Could you check a few things on this model? Use its own coordinates, in mm. Face numbers are marked on the shaded views. A direction names the side the tool comes from. Round coordinates to 2 decimals unless told otherwise and drop trailing zeros. Loops run counter-clockwise (first coordinate to the right, second up) from the corner with the lowest first, then second, coordinate; pieces in that order, holes last. Notation, with made-up numbers: (29, 39.25) -> (85, 39.25) arc R6 ccw to (85, 44.25) -> close; hole circle Ø2 at (55.25, 60.25). An arc over 180 degrees is marked (long way). One line per item, written item: value.
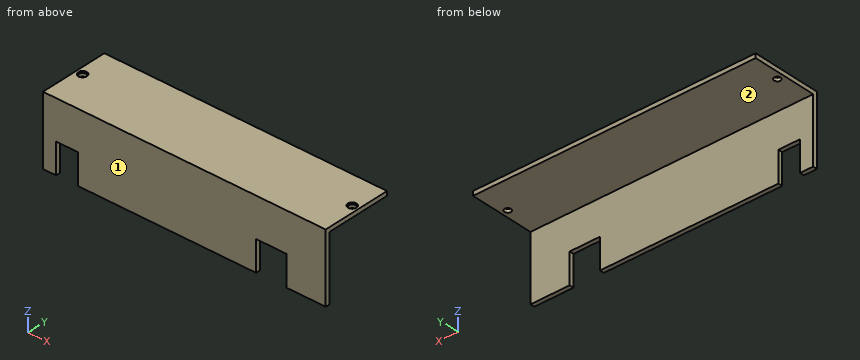
```python
from build123d import *

# Parameters (mm, degrees)
SKETCH021_W         = 130
SKETCH021_H         = 32
PAD009_DEPTH        = 2
HOLE005_D           = 3
HOLE005_DEPTH       = 25
HOLE005_CBORE_D     = 4
HOLE005_CBORE_DEPTH = 0.5
SKETCH023_W         = 130
SKETCH023_H         = 2
PAD010_DEPTH        = 30
SKETCH024_W         = 10
SKETCH024_H         = 15
SKETCH024_W_2       = 14
POCKET004_DEPTH     = 5


with BuildPart() as part:
    # Sketch021 → Pad009 (new body)
    with BuildSketch(Plane.XY.offset(31)):
        with Locations((65, -146.25)):
            Rectangle(SKETCH021_W, SKETCH021_H)
    extrude(amount=PAD009_DEPTH)

    # Hole005
    with Locations(Plane.XY.offset(33)):
        with Locations((3, -145), (127, -145)):
            CounterBoreHole(HOLE005_D / 2, HOLE005_CBORE_D / 2, HOLE005_CBORE_DEPTH, depth=HOLE005_DEPTH)

    # Sketch023 (on Face4 of Hole005) → Pad010 (join)
    with BuildSketch(Plane(origin=(0, 0, 31), x_dir=(1, 0, 0), z_dir=(0, 0, -1))):
        with Locations((65, 161.25)):
            Rectangle(SKETCH023_W, SKETCH023_H)
    extrude(amount=PAD010_DEPTH)

    # Sketch024 (on Face14 of Pad010) → Pocket004 (cut)
    with BuildSketch(Plane.XZ.offset(162.25)):
        with Locations((11, 7.5)):
            Rectangle(SKETCH024_W, SKETCH024_H)
        with Locations((105, 7.5)):
            Rectangle(SKETCH024_W_2, SKETCH024_H)
    extrude(amount=-POCKET004_DEPTH, mode=Mode.SUBTRACT)


solid = part.part
```
(1) On a 3-axis mill with a long thin cutter (end or side, diameter ignored), from which of +Z, -Z, +X, -X, +Y, -Y can I reach the whole of each face in a straight line? I mean the marked faces 1 and 2. Say none if no direction works.
Results below:
face 1: +Z, -Z, +X, -X, -Y
face 2: -Z, +X, -X, +Y
(2) Imagine slicing it at B-B on x = 127. Write out the boundary of the cut face in (y, z).
Results below:
outline: (-162.25, 1) -> (-160.25, 1) -> (-160.25, 31) -> (-146.5, 31) -> (-146.5, 32.5) -> (-147, 32.5) -> (-147, 33) -> (-162.25, 33) -> close; (-143.5, 31) -> (-130.25, 31) -> (-130.25, 33) -> (-143, 33) -> (-143, 32.5) -> (-143.5, 32.5) -> close
(3) Imagine slicing it at A-A on y = -145. Write out the boundary of the cut face in (x, z).
Results below:
outline: (0, 31) -> (1.5, 31) -> (1.5, 32.5) -> (1, 32.5) -> (1, 33) -> (0, 33) -> close; (4.5, 31) -> (125.5, 31) -> (125.5, 32.5) -> (125, 32.5) -> (125, 33) -> (5, 33) -> (5, 32.5) -> (4.5, 32.5) -> close; (128.5, 31) -> (130, 31) -> (130, 33) -> (129, 33) -> (129, 32.5) -> (128.5, 32.5) -> close
(4) Imagine slicing it at C-C on z = 11. Write out the boundary of the cut face in (x, y).
Results below:
outline: (0, -162.25) -> (6, -162.25) -> (6, -160.25) -> (0, -160.25) -> close; (16, -162.25) -> (98, -162.25) -> (98, -160.25) -> (16, -160.25) -> close; (112, -162.25) -> (130, -162.25) -> (130, -160.25) -> (112, -160.25) -> close
(5) For pin 1 Ø8 at (x, y) = (38, -150.5) entering from -Z; pin 2 Ø1 at (x, y) = (106.5, -161.5) entering from -Z; pin 3 Ø10 at (x, z) = (47.5, 19) entering from +Y, each with a flat end and sliding along its axis, tell me the tip position at first contact or that it passes through.
Results below:
pin 1: stops at z = 31
pin 2: stops at z = 15
pin 3: stops at y = -160.25
(6) Imagine slicing it at D-D on x = 85.5. Write out the boundary of the cut face in (y, z).
Results below:
outline: (-162.25, 1) -> (-160.25, 1) -> (-160.25, 31) -> (-130.25, 31) -> (-130.25, 33) -> (-162.25, 33) -> close
(7) Please list where these lines run through material, in increasing order: L1, parallel to X at y = -145, z = 31.8; L2, parallel to X at y = -145, z = 32.75; L3, parallel to Y at x = 127, z = 31.8.
Results below:
L1: x = 0 to 1.5, 4.5 to 125.5, 128.5 to 130
L2: x = 0 to 1, 5 to 125, 129 to 130
L3: y = -162.25 to -146.5, -143.5 to -130.25
